Source: CAD feature listing. Evaluate the final solid. Frame: model axes, mm. A direction names the side the tool comes from. Coordinates: 2 decimals unless noted, no trailing zeros. Loops run counter-clockwise (first coordinate to the right, second up) from the corner with the lowest first, then second, coordinate; pieces in that order, holes last.
```python
from build123d import *

# Parameters (mm, degrees)
SKETCH3_R          = 3.81
CUT_EXTRUDE1_DEPTH = 19.05
CIRPATTERN1_COUNT  = 5


with BuildPart() as part:
    # Sketch1 → Revolve2 (revolve)
    with BuildSketch(Plane.XY):
        with BuildLine():
            Line((0, 110.13359097), (0, 36.858618068))
            Line((0, 36.858618068), (38.1, 36.858618068))
            Line((38.1, 36.858618068), (38.1, 43.208618068))
            Line((38.1, 43.208618068), (9.525, 50.865266242))
            Line((9.525, 50.865266242), (9.525, 92.854369894))
            Line((9.525, 92.854369894), (38.1, 100.511018068))
            Line((38.1, 100.511018068), (38.1, 118.38859097))
            ThreePointArc((38.1, 118.38859097), (37.356051224, 120.184642194), (35.56, 120.92859097))
            Line((35.56, 120.92859097), (34.29, 120.92859097))
            ThreePointArc((34.29, 120.92859097), (32.493948776, 120.184642194), (31.75, 118.38859097))
            Line((31.75, 118.38859097), (31.75, 110.13359097))
            Line((31.75, 110.13359097), (0, 110.13359097))
        make_face()
        with BuildLine():
            Line((-38.1, 43.208618068), (-38.1, 36.858618068))
            Line((-38.1, 36.858618068), (0, 36.858618068))
            Line((0, 36.858618068), (0, 110.13359097))
            Line((0, 110.13359097), (-31.75, 110.13359097))
            Line((-31.75, 110.13359097), (-31.75, 118.38859097))
            ThreePointArc((-31.75, 118.38859097), (-32.493948776, 120.184642194), (-34.29, 120.92859097))
            Line((-34.29, 120.92859097), (-35.56, 120.92859097))
            ThreePointArc((-35.56, 120.92859097), (-37.356051224, 120.184642194), (-38.1, 118.38859097))
            Line((-38.1, 118.38859097), (-38.1, 100.511018068))
            Line((-38.1, 100.511018068), (-9.525, 92.854369894))
            Line((-9.525, 92.854369894), (-9.525, 50.865266242))
            Line((-9.525, 50.865266242), (-38.1, 43.208618068))
        make_face()
    revolve(axis=Axis((104.96947807, 20.983618068, 0), (-1, 0, 0)))

    # Sketch3 → Cut-Extrude1 (cut)
    with BuildSketch(Plane(origin=(9.525, 0, 0), x_dir=(0, 0, -1), z_dir=(1, 0, 0))):
        with Locations((0, 65.433618068)):
            Circle(SKETCH3_R)
    cut_extrude1 = extrude(amount=-CUT_EXTRUDE1_DEPTH, mode=Mode.SUBTRACT)

    # CirPattern1: Cut-Extrude1 ×5 about axis
    cirpattern1_axis = Axis((0, 20.983618068, 0), (1, 0, 0))
    for i in range(1, CIRPATTERN1_COUNT):
        add(cut_extrude1.rotate(cirpattern1_axis, i * 360 / CIRPATTERN1_COUNT), mode=Mode.SUBTRACT)


solid = part.part
```
Q1. First-contact query: pin 1 Ø8 at (x, y) = (2, 53) entering from -Z; pin 2 Ø3 at (x, y) = (-21, -56) entering from -Z; pin 3 Ø6 at (x, z) = (-26.5, -62.5) entering from -Y; pin 4 Ø7 at (y, z) = (65.43, 0) entering from -X. Flat tips, straight axial feed; report the tip coordinate or a pass-through.
Q2. Section query C-C on x = -1. Return the cut outline in (y, z) (3 decimals), then the cut area to 3 significant figures.
Q3. Section query B-B on z = 0. Count the separate pieces of the cut face and the enclosed holes in it, then the cut area to 3 significant figures.
Q4. Material intervals for line 1 along Y through (x, z) = (-9, 0); line 2 along Z through (x, y) = (13, 41.5); line 3 along Y through (x, z) = (22, -22), sorted ascending.
Q5. Draft query along Z for faces 1 (the flat face through (-38.1, 31, 15)), 2 (the conical face through (29.96, 32.25, 21.65)), 3 (the cylindrical face through (-0.4, -49.8, 54.2)). Return one class per face: released by +Z, released by -Z, zero draft, split by the parting line, or undercut.
Q6. Section query A-A on x = 22. Return the cut outline in (y, z) (3 decimals), then the cut area to 3 significant figures.
Q7. Reachability of faces 4 (the cylindrical face through (0.13, -18.04, -23.86)), 5 (the flat face through (9.525, 22, 31)), 6 (the flat face through (-31.75, -58, 43)) from +Z, -Z, +X, -X, +Y, -Y: full face, straight path, thin tool, end or side. Return the list, or none.
Resolved:
1. pin 1: stops at z = -84.63
1. pin 2: stops at z = -47.43
1. pin 3: stops at y = -45.41
1. pin 4: passes through
2. outline: circle Ø178.3 at (20.984, 0); hole circle Ø7.62 at (-14.977, -26.127); hole circle Ø7.62 at (-14.977, 26.127); hole circle Ø31.75 at (20.984, 0); hole circle Ø7.62 at (34.719, -42.274); hole circle Ø7.62 at (34.719, 42.274); hole circle Ø7.62 at (65.434, 0)
2. area: 23,900 mm2
3. separate pieces: 3
3. enclosed holes: 0
3. area: 5,610 mm2
4. line 1: y = -68.17 to 5.11, 36.86 to 61.62, 69.24 to 110.13
4. line 2: z = -86.76 to -69.85, -20.43 to 20.43, 69.85 to 86.76
4. line 3: y = -65.41 to -50.94, 6.14 to 35.83, 92.91 to 107.38
5. face 1: zero draft
5. face 2: undercut
5. face 3: split by the parting line
6. outline: circle Ø178.3 at (20.984, 0); circle Ø53.078 at (20.984, 0); hole circle Ø150.427 at (20.984, 0); hole circle Ø31.75 at (20.984, 0)
6. area: 8,620 mm2
7. face 4: +X, -X
7. face 5: +X
7. face 6: none
